Can you work these out from the model? Positions are in its coordinate system, mm. A direction names the side the tool comes from. Coordinates: 2 decimals unless noted, no trailing zeros. Write each loop counter-clockwise with the first axis right and the second up, starting at its lowest first coordinate (ties: lowest second). Pieces come first, ordered by that corner, then holes. Notation, with made-up numbers: (75, 43) -> (126, 43) arc R16 ccw to (126, 64) -> close; hole circle Ø11 at (9, 56). An arc over 180 degrees is marked (long way). Answer as CSV lines item,"result". Start each with the question number.
```python
from build123d import *

# Parameters (mm, degrees)
SKETCH1_R           = 6.35
BOSS_EXTRUDE1_DEPTH = 8.001
SKETCH1_3_R         = 7.366
SKETCH1_3_R_2       = 6.35
BOSS_EXTRUDE2_DEPTH = 1.143


with BuildPart() as part:
    # Sketch1 → Boss-Extrude1 (new body)
    with BuildSketch(Plane(origin=(0, 0, 0), x_dir=(1, 0, 0), z_dir=(0, 1, 0))):
        Circle(SKETCH1_R)
    extrude(amount=BOSS_EXTRUDE1_DEPTH)

    # Sketch1_3 → Boss-Extrude2 (add)
    with BuildSketch(Plane(origin=(0, 0, 0), x_dir=(1, 0, 0), z_dir=(0, 1, 0))):
        Circle(SKETCH1_3_R)
        Circle(SKETCH1_3_R_2, mode=Mode.SUBTRACT)
    extrude(amount=BOSS_EXTRUDE2_DEPTH)

    # Sketch3 one side → Revolve1 (revolve)
    with BuildSketch(Plane.XY):
        with BuildLine():
            Line((3.596294389, 0), (0, 0))
            Line((0, 0), (0, -2))
            ThreePointArc((0, -2), (2.057506582, -1.466366354), (3.596294389, 0))
        make_face()
    revolve(axis=Axis((0, 0, 0), (0, -1, 0)))


solid = part.part
```
Q1. Imagine slicing it at A-A (z = 0). Write out the boundary of the cut face in (x, y).
Q2. Imagine slicing it at B-B (x = 0). Write out the boundary of the cut face in (y, z).
Q3. For pin 1 (2 mm diameter, centred on x = -3, y = 2.5, fed in from +Z); pin 2 (1 mm diameter, centred on x = -2, y = 0, fed in from -Z); pin 3 (6 mm diameter, centred on y = 5.5, z = 1, fed in from -X), each with a flat end and sliding along its axis, tell me the tip position at first contact or that it passes through.
Q4. Which directions (+Z, -Z, +X, -X, +Y, -Y) give clear straight access to the entire face, cutting with the end or side of a thin tool? Please do faces 1 (the face through (-3.4, 0, -1.7)), 2 (the face through (0, 1.143, -7)), 3 (the face through (3.399, 0.563, 6.535)).
Q5. Imagine slicing it at D-D (z = -6). Write out the boundary of the cut face in (x, y).
Q6. Imagine slicing it at C-C (y = 3.5). Write out the boundary of the cut face in (x, z).
Q7. I need wall thicknesses on L1, parallel to Y at x = 0.5, z = 5.75; L2, parallel to X at y = 0.75, z = -0.25; L3, parallel to X at y = 5.25, z = 5.5. Which ranges of each line are inside material? Lowest first, please.
Entries:
1,outline,"(-7.37, 0) -> (-3.6, 0) arc R4.23 ccw to (3.6, 0) -> (7.37, 0) -> (7.37, 1.14) -> (6.35, 1.14) -> (6.35, 8) -> (-6.35, 8) -> (-6.35, 1.14) -> (-7.37, 1.14) -> close"
2,outline,"(0, -7.37) -> (1.14, -7.37) -> (1.14, -6.35) -> (8, -6.35) -> (8, 6.35) -> (1.14, 6.35) -> (1.14, 7.37) -> (0, 7.37) -> (0, 3.6) arc R4.23 ccw to (0, -3.6) -> close"
3,pin 1,"z = 6.03"
3,pin 2,"z = -7.21"
3,pin 3,"x = -6.35"
4,face 1,"-Y"
4,face 2,"+Y"
4,face 3,"+Y, -Y"
5,outline,"(-4.27, 0) -> (4.27, 0) -> (4.27, 1.14) -> (2.08, 1.14) -> (2.08, 8) -> (-2.08, 8) -> (-2.08, 1.14) -> (-4.27, 1.14) -> close"
6,outline,"circle Ø12.7 at (0, 0)"
7,L1,"0 to 8"
7,L2,"-7.36 to 7.36"
7,L3,"-3.17 to 3.17"
